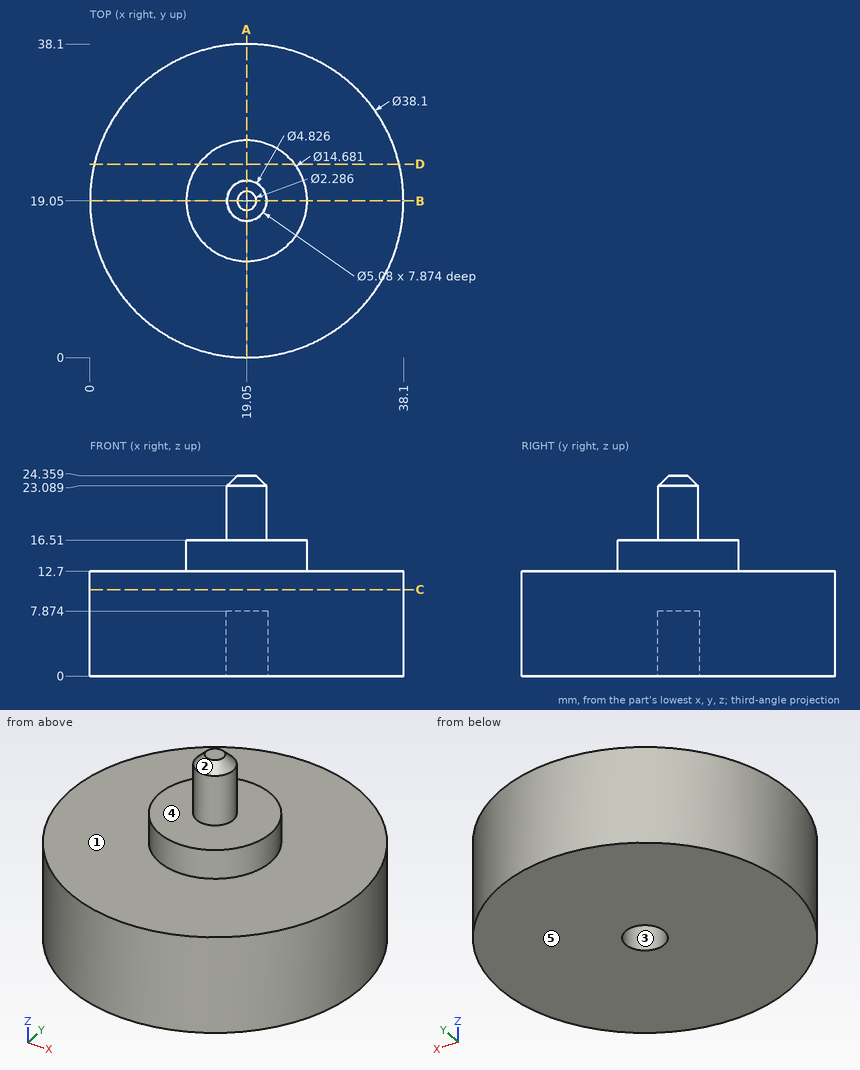
Answer from the drawing. Dimensions are ordinates in mm from the lowest x, y and z of the part. A direction names the side the tool comes from. Give positions to 0.01 mm unless a question says otherwise; leave off trailing zeros. Order: outer loops, then holes, each group sorted by start corner. A loop starts at its lowest first (then second) coordinate and runs counter-clockwise, first axis right, second up.
Item 1: The part is cut by section C-C, the plane z = 10.5. Give the vertices of the cut face in (x, y).
From the geometry:
outline: circle Ø38.1 at (19.05, 19.05)
Item 2: Given pin 1 Ø4 at (x, z) = (4.5, 7) entering from +Y; pin 2 Ø5 at (y, z) = (10.5, 13.5) entering from +X; pin 3 Ø5 at (x, y) = (22, 24.5) entering from +Z, each flat-ended and moving along its own axis, determine where each tip first touches the part or whether it passes through.
From the geometry:
pin 1: stops at y = 33.38
pin 2: stops at x = 37.07
pin 3: stops at z = 16.51
Item 3: For a pull along Y with two mould halves and no side action, classify the marked faces 1, 2 and 3 as pulls with the +Y half, pulls with the -Y half, needs draft (parallel to the pull), parting line crosses it, or undercut.
From the geometry:
face 1: needs draft
face 2: parting line crosses it
face 3: undercut
Item 4: The part is cut by section D-D, the plane y = 23.5. Give the vertices of the cut face in (x, z), and give its area (3 significant figures).
From the geometry:
outline: (0.53, 0) - (37.57, 0) - (37.57, 12.7) - (24.89, 12.7) - (24.89, 16.51) - (13.21, 16.51) - (13.21, 12.7) - (0.53, 12.7) - close
area: 515 mm2
Item 5: Find the intervals of material crossed by probe 1 along Y at (x, z) = (19.05, 5.25); probe 2 along Z at (x, y) = (17.5, 30); probe 3 along X at (y, z) = (19.5, 8) (1 decimal), in increasing order.
From the geometry:
probe 1: y = 0 to 16.51, 21.59 to 38.1
probe 2: z = 0 to 12.7
probe 3: x = 0 to 38.1
Item 6: Which of the six approach directions +Z, -Z, +X, -X, +Y, -Y give full straight-line access (tool end or side, diameter ignored) to the marked faces 4 and 5?
From the geometry:
face 4: +Z
face 5: -Z, +X, -X, +Y, -Y
Item 7: The part is cut by section A-A, the plane x = 19.05. Give the vertices of the cut face in (y, z).
From the geometry:
outline: (0, 0) - (16.51, 0) - (16.51, 7.87) - (21.59, 7.87) - (21.59, 0) - (38.1, 0) - (38.1, 12.7) - (26.39, 12.7) - (26.39, 16.51) - (21.46, 16.51) - (21.46, 23.09) - (20.19, 24.36) - (17.91, 24.36) - (16.64, 23.09) - (16.64, 16.51) - (11.71, 16.51) - (11.71, 12.7) - (0, 12.7) - close
